Source: CAD feature listing. Evaluate the final solid. Frame: model axes, mm. Face numbers are marked on the shaded views. A direction names the side the tool comes from. Give positions to 0.01 mm unless a question says otherwise; leave off trailing zeros. Order: outer loops, then holes, each group sorted by start corner. A loop starts at its lowest first (then second) coordinate and runs counter-clockwise, first axis right, second up.
from build123d import *


with BuildPart() as screw:
    # Sketch003 → Revolve (revolve)
    with BuildSketch(Plane.YZ):
        Polygon((0, 0), (1.6, 0), (1.6, 1), (3.2, 2.6), (3.2, 15), (0, 15), align=None)
    revolve(axis=Axis((0, 0, 0), (0, 0, 1)))


with BuildPart() as cut:
    # Sketch → Revolve001 (revolve)
    with BuildSketch(Plane.YZ):
        Polygon((3, 1.5), (7.5, 1.5), (7.5, 14.5), (6.7, 14.5), (6.7, 3.85), (5.35, 2.5), (4, 3.85), (4, 14.5), (0, 14.5), (0, 0), (1.5, 0), align=None)
    revolve(axis=Axis((0, 0, 0), (0, 0, 1)))

    # Cut: cut Screw
    add(screw.part, mode=Mode.SUBTRACT)


solid = cut.part
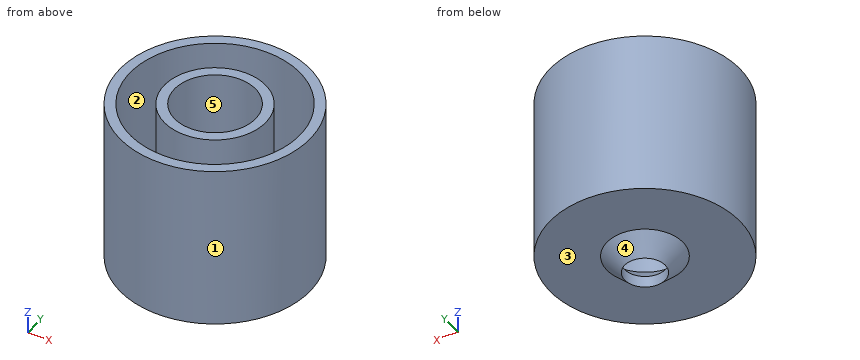
1) Section query A-A on x = 0. Output: boundary loops of the cut face in (y, z).
Checks:
outline: (-7.5, 1.5) - (-3, 1.5) - (-1.6, 0.1) - (-1.6, 1) - (-3.2, 2.6) - (-3.2, 14.5) - (-4, 14.5) - (-4, 3.85) - (-5.35, 2.5) - (-6.7, 3.85) - (-6.7, 14.5) - (-7.5, 14.5) - close; (1.6, 0.1) - (3, 1.5) - (7.5, 1.5) - (7.5, 14.5) - (6.7, 14.5) - (6.7, 3.85) - (5.35, 2.5) - (4, 3.85) - (4, 14.5) - (3.2, 14.5) - (3.2, 2.6) - (1.6, 1) - close
2) Reachability of the marked faces 1 and 2 from +Z, -Z, +X, -X, +Y, -Y: full face, straight path, thin tool, end or side. Return the list, or none.
Checks:
face 1: +Z, -Z
face 2: +Z
3) Ray query, L1, parallel to X at y = 0, z = 7; L2, parallel to X at y = -1, z = 5. Return the intervals inside material, ascending.
Checks:
L1: x = -7.5 to -6.7, -4 to -3.2, 3.2 to 4, 6.7 to 7.5
L2: x = -7.43 to -6.62, -3.87 to -3.04, 3.04 to 3.87, 6.62 to 7.43
4) First-contact query: pin 1 Ø4 at (x, z) = (-5, 11) entering from -Y; pin 2 Ø6 at (x, z) = (4, 9) entering from -Y; pin 3 Ø1.9 at (x, y) = (0, 0) entering from -Z; pin 4 Ø2 at (x, z) = (-2, 8) entering from +Y. Flat tips, straight axial feed; report the tip coordinate or a pass-through.
Checks:
pin 1: stops at y = -6.87
pin 2: stops at y = -7.43
pin 3: passes through
pin 4: stops at y = 7.43
5) Section query C-C on z = 7.75. Output: boundary loops of the cut face in (x, y).
Checks:
outline: circle Ø15 at (0, 0); circle Ø8 at (0, 0); hole circle Ø13.4 at (0, 0); hole circle Ø6.4 at (0, 0)
6) Pull-direction query (Y, two-part tool) for the marked faces 3, 4 and 5; classes: +Y half, -Y half, draft (parallel to the pull), parting line (faces both ways), or undercut.
Checks:
face 3: draft
face 4: parting line
face 5: undercut
